Verification items for the finished model (mm, model axes). Face numbers are marked on the shaded views. A direction names the side the tool comes from. Coordinates: 2 decimals unless noted, no trailing zeros. Loops run counter-clockwise (first coordinate to the right, second up) from the corner with the lowest first, then second, coordinate; pieces in that order, holes last.
Q1. Mould release check, pull along X, two halves, no side actions. Record for the marked faces 3, 4 and 5: +X half, -X half, draft (parallel to the pull), parting line (faces both ways), or undercut.
Q2. Sectioned sample at B-B (y = 21.5). Enter the section's corners in (x, z).
Q3. Access from +Z, -Z, +X, -X, +Y, -Y to the whole of each face (thin tool, end or side, straight path). Record for the marked faces 1 and 2.
Q4. Go/stop test with flat-tipped pins: P1, Ø0.8, axis at y = 67, z = -99, coming from the -X side; P2, Ø8, axis at x = 24.5, z = -6, coming from the +Y side; P3, Ø5.5, axis at x = 98.5, z = 9.5, coming from the +Y side. Record where each tip stops, or that it passes through.
Q5. Material ranges on probe 1 along Z at (x, y) = (75.5, 66); probe 2 along X at (y, z) = (10, 64.5), recorded low to high.
Q6. Sectioned sample at A-A (z = 85.5). Enter the section's corners in (x, y).
Q7. Sectioned sample at C-C (x = -64). Enter the section's corners in (y, z), then the cut area to 3 significant figures.
Q8. Sectioned sample at D-D (z = -4). Enter the section's corners in (x, y).
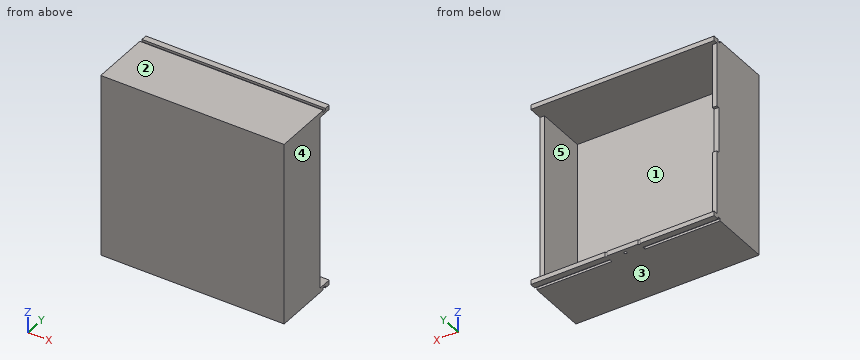
```python
from build123d import *

# Parameters (mm, degrees)
SKETCH_1_W               = 200
SKETCH_1_H               = 200
EXTRUDE_2_DEPTH          = 5
SKETCH_2_W               = 200
SKETCH_2_H               = 5
EXTRUDE_3_DEPTH          = 70
SKETCH_3_W               = 5
SKETCH_3_H               = 190
EXTRUDE_4_DEPTH          = 54.7
SKETCH_4_W               = 200
SKETCH_4_H               = 5
EXTRUDE_5_DEPTH          = 70
SKETCH_14_W              = 5
SKETCH_14_H              = 190
EXTRUDE_7_DEPTH          = 65.3
SKETCH_15_W              = 5
SKETCH_15_H              = 50
CUT_EXTRUDE_7_DEPTH      = 3
CUT_EXTRUDE_8_DEPTH      = 1
CUT_EXTRUDE_8_DEPTH_BACK = 5
CUT_EXTRUDE_9_DEPTH      = 1
CUT_EXTRUDE_9_DEPTH_BACK = 5
SKETCH_19_R              = 1.5
CUT_EXTRUDE_10_DEPTH     = 5
SKETCH_20_W              = 200
SKETCH_20_H              = 3.5
CUT_EXTRUDE_11_DEPTH     = 2.5
SKETCH_21_W              = 82
SKETCH_21_H              = 3.5
CUT_EXTRUDE_13_DEPTH     = 2.5


with BuildPart() as part:
    # Эскиз1 → Бобышка-Вытянуть2 (new body)
    with BuildSketch(Plane(origin=(0, 0, 0), x_dir=(1, 0, 0), z_dir=(0, 1, 0))):
        Rectangle(SKETCH_1_W, SKETCH_1_H)
    extrude(amount=EXTRUDE_2_DEPTH)

    # Эскиз2 → Бобышка-Вытянуть3 (add)
    with BuildSketch(Plane(origin=(0, 5, 0), x_dir=(1, 0, 0), z_dir=(0, 1, 0))):
        with Locations((0, -97.5)):
            Rectangle(SKETCH_2_W, SKETCH_2_H)
    extrude(amount=EXTRUDE_3_DEPTH)

    # Эскиз3 → Бобышка-Вытянуть4 (add)
    with BuildSketch(Plane(origin=(0, 5, 0), x_dir=(1, 0, 0), z_dir=(0, 1, 0))):
        with Locations((97.5, 0)):
            Rectangle(SKETCH_3_W, SKETCH_3_H)
    extrude(amount=EXTRUDE_4_DEPTH)

    # Эскиз4 → Бобышка-Вытянуть5 (add)
    with BuildSketch(Plane(origin=(0, 5, 0), x_dir=(1, 0, 0), z_dir=(0, 1, 0))):
        with Locations((0, 97.5)):
            Rectangle(SKETCH_4_W, SKETCH_4_H)
    extrude(amount=EXTRUDE_5_DEPTH)

    # Эскиз14 → Бобышка-Вытянуть7 (add)
    with BuildSketch(Plane(origin=(0, 5, 0), x_dir=(1, 0, 0), z_dir=(0, 1, 0))):
        with Locations((-97.5, 0)):
            Rectangle(SKETCH_14_W, SKETCH_14_H)
    extrude(amount=EXTRUDE_7_DEPTH)

    # Эскиз15 → Вырез-Вытянуть7 (cut)
    with BuildSketch(Plane(origin=(0, 70.3, 0), x_dir=(1, 0, 0), z_dir=(0, 1, 0))):
        with Locations((-97.5, 0)):
            Rectangle(SKETCH_15_W, SKETCH_15_H)
    extrude(amount=-CUT_EXTRUDE_7_DEPTH, mode=Mode.SUBTRACT)

    # Эскиз16 → Вырез-Вытянуть8 (cut, two sides)
    with BuildSketch(Plane(origin=(0, 0, -100), x_dir=(-1, 0, 0), z_dir=(0, 0, -1))) as cut_extrude_8_sk:
        with BuildLine():
            Line((-19, 366.325434328), (-19, 75))
            ThreePointArc((-19, 75), (-18, 74), (-17, 75))
            Line((-17, 75), (-17, 366.325434328))
            Line((-17, 366.325434328), (-17, 948.976302985))
            Line((-17, 948.976302985), (-19, 948.976302985))
            Line((-19, 948.976302985), (-19, 366.325434328))
        make_face()
    extrude(amount=CUT_EXTRUDE_8_DEPTH, mode=Mode.SUBTRACT)
    extrude(cut_extrude_8_sk.sketch, amount=-CUT_EXTRUDE_8_DEPTH_BACK, mode=Mode.SUBTRACT)

    # Эскиз18 → Вырез-Вытянуть9 (cut, two sides)
    with BuildSketch(Plane(origin=(0, 0, -100), x_dir=(-1, 0, 0), z_dir=(0, 0, -1))) as cut_extrude_9_sk:
        with BuildLine():
            Line((17, 366.325434328), (17, 75))
            ThreePointArc((17, 75), (18, 74), (19, 75))
            Line((19, 75), (19, 366.325434328))
            Line((19, 366.325434328), (19, 948.976302985))
            Line((19, 948.976302985), (17, 948.976302985))
            Line((17, 948.976302985), (17, 366.325434328))
        make_face()
    extrude(amount=CUT_EXTRUDE_9_DEPTH, mode=Mode.SUBTRACT)
    extrude(cut_extrude_9_sk.sketch, amount=-CUT_EXTRUDE_9_DEPTH_BACK, mode=Mode.SUBTRACT)

    # Эскиз19 → Вырез-Вытянуть10 (cut)
    with BuildSketch(Plane(origin=(0, 0, -100), x_dir=(-1, 0, 0), z_dir=(0, 0, -1))):
        with Locations((0, 70)):
            Circle(SKETCH_19_R)
    extrude(amount=-CUT_EXTRUDE_10_DEPTH, mode=Mode.SUBTRACT)

    # Эскиз20 → Вырез-Вытянуть11 (cut)
    with BuildSketch(Plane.XY.offset(100)):
        with Locations((0, 66.75)):
            Rectangle(SKETCH_20_W, SKETCH_20_H)
    extrude(amount=-CUT_EXTRUDE_11_DEPTH, mode=Mode.SUBTRACT)

    # Эскиз21 → Вырез-Вытянуть13 (cut)
    with BuildSketch(Plane(origin=(0, 0, -100), x_dir=(-1, 0, 0), z_dir=(0, 0, -1))):
        with Locations((-59, 66.75)):
            Rectangle(SKETCH_21_W, SKETCH_21_H)
        with Locations((59, 66.75)):
            Rectangle(SKETCH_21_W, SKETCH_21_H)
    extrude(amount=-CUT_EXTRUDE_13_DEPTH, mode=Mode.SUBTRACT)


solid = part.part
```
Geometry check:
1. face 3: draft
1. face 4: +X half
1. face 5: undercut
2. outline: (-100, -100) - (100, -100) - (100, 100) - (-100, 100) - close; hole (-95, -95) - (95, -95) - (95, 95) - (-95, 95) - close
3. face 1: +Y
3. face 2: +Z, +X, -X, +Y, -Y
4. P1: stops at x = -18
4. P2: stops at y = 5
4. P3: stops at y = 59.7
5. probe 1: z = -97.5 to -95, 95 to 97.5
5. probe 2: x = -100 to -95, 95 to 100
6. outline: (-100, 0) - (100, 0) - (100, 59.7) - (95, 59.7) - (95, 5) - (-95, 5) - (-95, 70.3) - (-100, 70.3) - close
7. outline: (0, -100) - (65, -100) - (65, -97.5) - (68.5, -97.5) - (68.5, -100) - (75, -100) - (75, -95) - (5, -95) - (5, 95) - (75, 95) - (75, 100) - (68.5, 100) - (68.5, 97.5) - (65, 97.5) - (65, 100) - (0, 100) - close
7. area: 1,680 mm2
8. outline: (-100, 0) - (100, 0) - (100, 59.7) - (95, 59.7) - (95, 5) - (-95, 5) - (-95, 67.3) - (-100, 67.3) - close
